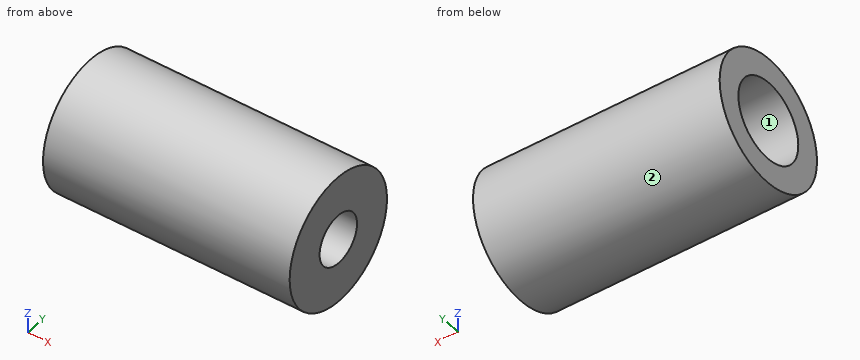
from build123d import *

# Parameters (mm, degrees)
SKETCH1_R           = 6.5
BOSS_EXTRUDE1_DEPTH = 12.5
SKETCH2_R           = 2.5
CUT_EXTRUDE1_DEPTH  = 12.5
SKETCH3_R           = 4
CUT_EXTRUDE2_DEPTH  = 12.5


with BuildPart() as part:
    # Sketch1 → Boss-Extrude1 (new, symmetric)
    with BuildSketch(Plane(origin=(0, 0, 0), x_dir=(0, 0, -1), z_dir=(1, 0, 0))):
        Circle(SKETCH1_R)
    extrude(amount=BOSS_EXTRUDE1_DEPTH, both=True)

    # Sketch2 → Cut-Extrude1 (cut)
    with BuildSketch(Plane(origin=(12.5, 0, 0), x_dir=(0, 0, -1), z_dir=(1, 0, 0))):
        Circle(SKETCH2_R)
    extrude(amount=-CUT_EXTRUDE1_DEPTH, mode=Mode.SUBTRACT)

    # Sketch3 → Cut-Extrude2 (cut)
    with BuildSketch(Plane.ZY.offset(12.5)):
        Circle(SKETCH3_R)
    extrude(amount=-CUT_EXTRUDE2_DEPTH, mode=Mode.SUBTRACT)


solid = part.part
Work out the finished part from the listing and answer in its coordinate system (mm). Face numbers are marked on the shaded views. A direction names the side the tool comes from. Give positions to 0.01 mm unless a question says otherwise; leave off trailing zeros. Loops run counter-clockwise (first coordinate to the right, second up) from the corner with the lowest first, then second, coordinate; pieces in that order, holes last. Notation, with made-up numbers: (-2.75, -21) - (37.25, -21) arc R15 cw to (37.25, 5) - close; hole circle Ø7 at (19.25, -24.5). An arc over 180 degrees is marked (long way). Answer in a Markdown table with one row per item.
(1) Section C-C (x = -8) is taken. Give the vertices of the cut face in (y, z).
Results list:
| item | result |
|---|---|
| outline | circle Ø13 at (0, 0); hole circle Ø8 at (0, 0) |
(2) Section D-D (y = -3.5) is taken. Give the vertices of the cut face in (x, z).
Results list:
| item | result |
|---|---|
| outline | (-12.5, -5.48) - (12.5, -5.48) - (12.5, 5.48) - (-12.5, 5.48) - (-12.5, 1.94) - (0, 1.94) - (0, -1.94) - (-12.5, -1.94) - close |
(3) Consider L1, parallel to Y at x = -8.75, z = 0; L2, parallel to Y at x = 7, z = 0; L3, parallel to X at y = 2.5, z = 2.5. Determine where each line is inside the solid, lowest interval first. Write a range as [from, to].
Results list:
| item | result |
|---|---|
| L1 | y = [-6.5, -4], [4, 6.5] |
| L2 | y = [-6.5, -2.5], [2.5, 6.5] |
| L3 | x = [0, 12.5] |
(4) A tool of negligible diameter and unlimited length cuts with its end or side. For the marked faces 1 and 2, from which of +Z, -Z, +X, -X, +Y, -Y can it reach the whole face along a straight path? Write none if from no direction.
Results list:
| item | result |
|---|---|
| face 1 | -X |
| face 2 | +X, -X |
(5) Section A-A (y = 0) is taken. Give the vertices of the cut face in (x, z).
Results list:
| item | result |
|---|---|
| outline | (-12.5, -6.5) - (12.5, -6.5) - (12.5, -2.5) - (0, -2.5) - (0, -4) - (-12.5, -4) - close; (-12.5, 4) - (0, 4) - (0, 2.5) - (12.5, 2.5) - (12.5, 6.5) - (-12.5, 6.5) - close |
(6) Flat-ended cylindrical pins translate along their axes: pin 1 Ø3 at (x, y) = (4.5, -4) entering from +Z; pin 2 Ø5 at (x, y) = (-4, -3) entering from -Z; pin 3 Ø4 at (y, z) = (-1.5, 0.5) entering from -X. Find the tip coordinate at first contact, or state that the pin passes through.
Results list:
| item | result |
|---|---|
| pin 1 | stops at z = 6 |
| pin 2 | stops at z = -6.48 |
| pin 3 | stops at x = 0 |
